Can you work these out from the model? Positions are in its coordinate system, mm. A direction names the side the tool comes from. Give positions to 0.01 mm unless a question says otherwise; leave off trailing zeros. Write each loop counter-clockwise with the first axis right and the second up, starting at its lowest first coordinate (ties: lowest second). Pieces come first, ordered by that corner, then holes. Notation, with made-up numbers: M -18,8 L 28,8 A19 cw 28,45 Z; hole C 23,-14.75 d9. An arc over 180 degrees is marked long. Write each question's results on one line, items separated by ' | '.
from build123d import *

# Parameters (mm, degrees)
CUT_EXTRUDE10_DEPTH = 1.984375


with BuildPart() as part:
    # Sketch22 → Revolve1 (revolve)
    with BuildSketch(Plane(origin=(0, 0, 0), x_dir=(0, 0, -1), z_dir=(1, 0, 0)), mode=Mode.PRIVATE) as revolve1_sk:
        Polygon((-15.875, 0), (-15.875, 2.54), (-15.430368213, 3.175), (12.9794, 3.175), (14.1732, 1.9812), (15.875, 1.9812), (15.875, 0), align=None)
    revolve(revolve1_sk.sketch.rotate(Axis((0, 0, -15.875), (0, 0, 1)), 90), axis=Axis((0, 0, -15.875), (0, 0, 1)))

    # Sketch23 → Cut-Extrude10 (cut)
    with BuildSketch(Plane.XY.offset(15.875)):
        Polygon((0, 1.833087105), (-1.5875, 0.916543552), (-1.5875, -0.916543552), (0, -1.833087105), (1.5875, -0.916543552), (1.5875, 0.916543552), align=None)
    extrude(amount=-CUT_EXTRUDE10_DEPTH, mode=Mode.SUBTRACT)

    # Cut-Extrude11 cone 1 section (on through the dimple's axis) → Cut-Extrude11 (revolve, cut)
    with BuildSketch(Plane(origin=(0, 0, 15.875), x_dir=(0, -1, 0), z_dir=(1, 0, 0))):
        Polygon((0, 0), (1.833087105, 0), (0, 1.833087105), align=None)
    revolve(axis=Axis((0, 0, 15.875), (0, 0, -1)), mode=Mode.SUBTRACT)

    # Cut-Extrude12 cone 1 section (on through the dimple's axis) → Cut-Extrude12 (revolve, cut)
    with BuildSketch(Plane(origin=(0, 0, 13.890625), x_dir=(0, -1, 0), z_dir=(1, 0, 0))):
        Polygon((0, 0), (1.5875, 0), (0, 0.916543552), align=None)
    revolve(axis=Axis((0, 0, 13.890625), (0, 0, -1)), mode=Mode.SUBTRACT)


solid = part.part
Item 1: I want a section at A-A, the plane z = 12. Please give me the cut outline in (x, y) (3 decimals).
Geometry says:
outline: C 0,0 d6.35
Item 2: For faces 1 (the face through (1, 2, 15.875)), 2 (the face through (1.46, -1.34, -15.04)), 3 (the face through (0.8, 1.37, 14.9)), which set-ups out of +Z, -Z, +X, -X, +Y, -Y let a thin tool reach every point of the face, with its end or its side?
Geometry says:
face 1: +Z, +X, -X, +Y, -Y | face 2: -Z | face 3: +Z
Item 3: I'm going to push flat-ended pins straight in: pin 1 (0.5 mm diameter, centred on y = -0.5, z = 15.5, fed in from +X); pin 2 (1 mm diameter, centred on x = 1, z = 12, fed in from -Y). Where does each tip first touch, or does it pass through?
Geometry says:
pin 1: stops at x = 3.16 | pin 2: stops at y = -3.14
Item 4: If I drill on line 1 (X direction, y = 0.25, z = 14.5); line 2 (X direction, y = 1.5, z = 7); line 3 (Z direction, x = 2, y = -2), over which ranges is the centre line in solid material (lowest first)? Write a range as from..to.
Geometry says:
line 1: x = -3.17..-1.59, 1.59..3.17 | line 2: x = -2.8..2.8 | line 3: z = -13.33..15.67
Item 5: Thinking about a two-plate mould opening in X: for faces 4 (the face through (2.52, 1.93, 1.03)), 5 (the face through (0, 0, -15.875)), 6 (the face through (0.783, -1.381, 14.897)), which applies, +X half, -X half, draft (parallel to the pull), parting line (faces both ways), or undercut?
Geometry says:
face 4: parting line | face 5: draft | face 6: undercut
